```python
from build123d import *

# Parameters (mm, degrees)
EXTRUDE_1_DEPTH     = 42
SKETCH_2_R          = 15
CUT_EXTRUDE_1_DEPTH = 12
SKETCH_3_W          = 30
SKETCH_3_H          = 20
CUT_EXTRUDE_2_DEPTH = 8
SKETCH_4_W          = 5
SKETCH_4_H          = 8
EXTRUDE_2_DEPTH     = 3
OTHER_START         = 8
OTHER_1_OUTLINE_R   = 1.7
OTHER_1_DEPTH       = 34
SKETCH_7_W          = 20
SKETCH_7_H          = 32
CUT_EXTRUDE_6_DEPTH = 26
CUT_EXTRUDE_7_DEPTH = 60.699246226


# Read off the part's stored shape, not the designer's step: 高级异型孔1, 高级异型孔2
with BuildPart() as part:
    # 草图1 → 凸台-拉伸1 (new body)
    with BuildSketch(Plane.XY):
        with BuildLine():
            Line((0, 0), (5.769230769, -13.846153846))
            ThreePointArc((5.769230769, -13.846153846), (15, -20), (24.230769231, -13.846153846))
            Line((24.230769231, -13.846153846), (30, 0))
            Line((30, 0), (30, 30))
            Line((30, 30), (0, 30))
            Line((0, 30), (0, 0))
        make_face()
    extrude(amount=EXTRUDE_1_DEPTH)

    # 草图2 → 切除-拉伸1 (cut, symmetric)
    with BuildSketch(Plane(origin=(0, 0, 25), x_dir=(-1, 0, 0), z_dir=(0, 0, -1))):
        with Locations((-15, -10)):
            Circle(SKETCH_2_R)
    extrude(amount=CUT_EXTRUDE_1_DEPTH, both=True, mode=Mode.SUBTRACT)

    # 草图3 → 切除-拉伸2 (cut)
    with BuildSketch(Plane(origin=(0, 0, 0), x_dir=(-1, 0, 0), z_dir=(0, 0, -1))):
        with Locations((-15, -10)):
            Rectangle(SKETCH_3_W, SKETCH_3_H)
    extrude(amount=-CUT_EXTRUDE_2_DEPTH, mode=Mode.SUBTRACT)

    # 草图4 → 凸台-拉伸2 (add)
    with BuildSketch(Plane(origin=(0, 0, 0), x_dir=(-1, 0, 0), z_dir=(0, 0, -1))):
        with Locations((-27.5, 15)):
            Rectangle(SKETCH_4_W, SKETCH_4_H)
        with Locations((-2.5, 15)):
            Rectangle(SKETCH_4_W, SKETCH_4_H)
    extrude(amount=EXTRUDE_2_DEPTH)

    # 高级异型孔1 outline → 高级异型孔1 (cut)
    with BuildSketch(Plane.XY.offset(OTHER_START)):
        with Locations((15, -10)):
            Circle(OTHER_1_OUTLINE_R)
    extrude(amount=OTHER_1_DEPTH, mode=Mode.SUBTRACT)

    # 草图7 → 切除-拉伸6 (cut)
    with BuildSketch(Plane(origin=(0, 30, 0), x_dir=(1, 0, 0), z_dir=(0, 1, 0))):
        with Locations((15, -26)):
            Rectangle(SKETCH_7_W, SKETCH_7_H)
    extrude(amount=-CUT_EXTRUDE_6_DEPTH, mode=Mode.SUBTRACT)

    # 草图8 → 切除-拉伸7 (cut, through all)
    with BuildSketch(Plane(origin=(30, 0, 0), x_dir=(0, 0, -1), z_dir=(1, 0, 0))):
        Polygon((-42, 30), (-10, 30), (-42, 4), align=None)
    extrude(amount=-CUT_EXTRUDE_7_DEPTH, mode=Mode.SUBTRACT)

    # 高级异型孔2 outline → 高级异型孔2 (revolve, cut)
    with BuildSketch(Plane(origin=(15, 15, 0), x_dir=(1, 0, 0), z_dir=(0, -1, 0))):
        Polygon((0, 0), (1.7, 0), (1.7, 8.55), (3.15, 10), (0, 10), align=None)
    revolve(axis=Axis((15, 15, 0), (0, 0, 1)), mode=Mode.SUBTRACT)


solid = part.part
```
CAD build for the part. Positions are in the model's coordinates, mm. A direction names the side the tool comes from. Round coordinates to 2 decimals unless told otherwise and drop trailing zeros. Order: outer loops, then holes, each group sorted by start corner. A loop starts at its lowest first (then second) coordinate and runs counter-clockwise, first axis right, second up. Notation, with made-up numbers: (9, 65.5) - (13, 65.5) arc R28 ccw to (13, 99.5) - close; hole circle Ø2 at (-9.75, 7). An arc over 180 degrees is marked (long way). Answer in a Markdown table with one row per item. Add a question column.
(1) Mould opens along Z. For faces 1 (the face through (16.57, 14.35, 4.33)), 2 (the face through (15, -8, 13)), 3 (the face through (3, 17, 26)) say: +Z half, -Z half, draft (parallel to the pull), parting line (faces both ways), or undercut.
(2) Band-saw the part on A-A on x = 15. List the corners of the cut face in (y, z).
(3) Band-saw the part on B-B on z = 34. List the corners of the cut face in (x, y).
(4) Band-saw the part on D-D on y = -10. List the corners of the cut face in (x, z).
(5) Drop flat-ended pins along their axis: pin 1 Ø1.5 at (x, y) = (22.5, 19) entering from -Z; pin 2 Ø6 at (x, z) = (20, 20.5) entering from -Y; pin 3 Ø4 at (x, y) = (11.5, 7) entering from +Z. Give the stop position or say it passes through.
(6) Probe L1, parallel to Y at x = 15, z = 3.5; L2, parallel to Y at x = 15, z = 38.35; L3, parallel to Z at x = 7.25, y = -7. List the from-to ranges inside material, lowest first. Write a range as [from, to].
(7) 3-axis set-ups, long thin cutter, end or side, ignore diameter. For faces 4 (the face through (15, -20, 39)), 5 (the face through (15, -8, 37)), 6 (the face through (28, 19, -1)), 7 (the face through (5, 11, 19)), 8 (the face through (3, 11, -1)): which of +Z, -Z, +X, -X, +Y, -Y reach the whole face in a straight line?
(8) Band-saw the part on C-C on y = -4.5. List the corners of the cut face in (x, z) (3 decimals), and give its area (4 significant figures).
Data:
| question | item | result |
|---|---|---|
| 1 | face 1 | draft |
| 1 | face 2 | undercut |
| 1 | face 3 | +Z half |
| 2 | outline | (-20, 8) - (-11.7, 8) - (-11.7, 13) - (-20, 13) - close; (-20, 37) - (-11.7, 37) - (-11.7, 42) - (-20, 42) - close; (-8.3, 8) - (0, 8) - (0, 0) - (13.3, 0) - (13.3, 8.55) - (11.85, 10) - (4, 10) - (4, 13) - (-8.3, 13) - close; (-8.3, 37) - (4, 37) - (4, 42) - (-8.3, 42) - close; (16.7, 0) - (30, 0) - (30, 10) - (18.15, 10) - (16.7, 8.55) - close |
| 3 | outline | (0, 0) - (1.47, -3.53) arc R15 cw to (9.61, 4) - (5, 4) - (5, 10.5) - (0, 10.5) - close; (20.39, 4) arc R15 cw to (28.53, -3.53) - (30, 0) - (30, 10.5) - (25, 10.5) - (25, 4) - close |
| 4 | outline | (4.17, 8) - (13.3, 8) - (13.3, 13) - (4.17, 13) - close; (4.17, 37) - (13.3, 37) - (13.3, 42) - (4.17, 42) - close; (16.7, 8) - (25.83, 8) - (25.83, 13) - (16.7, 13) - close; (16.7, 37) - (25.83, 37) - (25.83, 42) - (16.7, 42) - close |
| 5 | pin 1 | stops at z = 0 |
| 5 | pin 2 | stops at y = 2.69 |
| 5 | pin 3 | stops at z = 10 |
| 6 | L1 | y = [0, 13.3], [16.7, 30] |
| 6 | L2 | y = [-20, -11.7], [-8.3, 4] |
| 6 | L3 | z = [8, 13], [37, 42] |
| 7 | face 4 | +Z, -Z, -Y |
| 7 | face 5 | -Y |
| 7 | face 6 | -Z, +X, -X, +Y |
| 7 | face 7 | +Z, +Y |
| 7 | face 8 | -Z, +X, -X, -Y |
| 8 | outline | (1.875, 8) - (28.125, 8) - (28.125, 13) - (1.875, 13) - close; (1.875, 37) - (28.125, 37) - (28.125, 42) - (1.875, 42) - close |
| 8 | area | 262.5 mm^2 |
